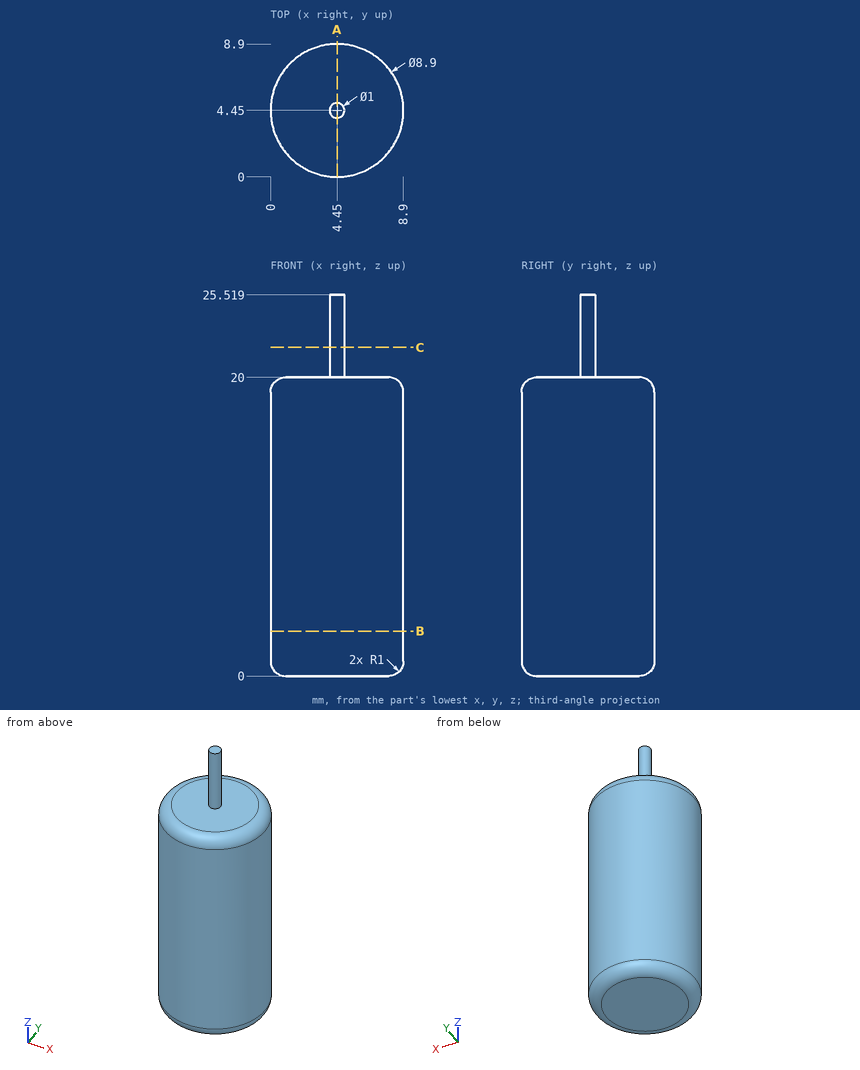
Check sheet for the drawn part. Datum: minimum x, y, z corner. Units: mm. Round coordinates to 2 decimals unless told otherwise and drop trailing zeros. Write each loop counter-clockwise with the first axis right and the second up, starting at its lowest first coordinate (ties: lowest second). Pieces come first, ordered by that corner, then holes. Notation, with made-up numbers: (53, 59) -> (58, 59) arc R34 ccw to (58, 98) -> close; hole circle Ø2 at (6, 52). An arc over 180 degrees is marked (long way). Write each question's results on one line, items separated by ' | '. Start each with the question number.
1. Cross-section at A-A (x = 4.45). Enter the section's corners in (y, z), then the cut area to 3 significant figures.
2. Material ranges on probe 1 along Z at (x, y) = (4, 5.75); probe 2 along X at (y, z) = (5.5, 5.5) (1 decimal); probe 3 along Z at (x, y) = (1, 2) (1 decimal), recorded low to high. Write a range as from..to.
3. Cross-section at C-C (z = 22). Enter the section's corners in (x, y).
4. Depth check by flat-ended pin: P1, Ø3, axis at x = 3.5, y = 1.5, coming from the +Z side; P2, Ø1, axis at y = 6, z = 8.5, coming from the -X side. Enter the tip coordinate at first touch or a pass-through.
5. Cross-section at B-B (z = 3). Enter the section's corners in (x, y).
Solutions:
1) outline: (0, 1) arc R1 ccw to (1, 0) -> (7.9, 0) arc R1 ccw to (8.9, 1) -> (8.9, 19) arc R1 ccw to (7.9, 20) -> (4.95, 20) -> (4.95, 25.52) -> (3.95, 25.52) -> (3.95, 20) -> (1, 20) arc R1 ccw to (0, 19) -> close | area: 183 mm2
2) probe 1: z = 0..20 | probe 2: x = 0.1..8.8 | probe 3: z = 0.4..19.6
3) outline: circle Ø1 at (4.45, 4.45)
4) P1: stops at z = 20 | P2: stops at x = 0.13
5) outline: circle Ø8.9 at (4.45, 4.45)
